Model file for the job. Use its own axes, mm. A direction names the side the tool comes from. Coordinates: 2 decimals unless noted, no trailing zeros. Loops run counter-clockwise (first coordinate to the right, second up) from the corner with the lowest first, then second, coordinate; pieces in that order, holes last.
from build123d import *

# Parameters (mm, degrees)
BASE_FLANGE1_DEPTH = 2
SKETCH7_R          = 2
CUT_EXTRUDE1_DEPTH = 2
SKETCH9_R          = 1.9431
CUT_EXTRUDE2_DEPTH = 2


# Sheet-metal steps are written as plain solids
with BuildPart() as part:
    # Sketch2 → Base-Flange1 (new body)
    with BuildSketch(Plane(origin=(0, 0, 0), x_dir=(1, 0, 0), z_dir=(0, 1, 0))):
        with BuildLine():
            Line((-26.055569119, -21.875), (-26.055569119, -46.875))
            Line((-26.055569119, -46.875), (-16.055569119, -46.875))
            Line((-16.055569119, -46.875), (-16.055569119, -21.875))
            Line((-16.055569119, -21.875), (26.055569119, -21.875))
            Line((26.055569119, -21.875), (26.055569119, 8.188046441))
            ThreePointArc((26.055569119, 8.188046441), (21.514872246, 4.669726518), (15.870079226, 5.73406431))
            ThreePointArc((15.870079226, 5.73406431), (10.616247764, 4.133629141), (7, 0))
            ThreePointArc((7, 0), (0, -7), (-7, 0))
            ThreePointArc((-7, 0), (-10.616247764, 4.133629141), (-15.870079226, 5.73406431))
            ThreePointArc((-15.870079226, 5.73406431), (-21.514872246, 4.669726518), (-26.055569119, 8.188046441))
            Line((-26.055569119, 8.188046441), (-26.055569119, -21.875))
        make_face()
    extrude(amount=-BASE_FLANGE1_DEPTH)

    # Sketch7 → Cut-Extrude1 (cut)
    with BuildSketch(Plane(origin=(0, 0, 0), x_dir=(1, 0, 0), z_dir=(0, 1, 0))):
        with Locations(Location((-21.055569119, -40.375, 0), (0, 0, 270))):
            Circle(SKETCH7_R)
        with Locations(Location((-21.055569119, -30.875, 0), (0, 0, 270))):
            Circle(SKETCH7_R)
    extrude(amount=-CUT_EXTRUDE1_DEPTH, mode=Mode.SUBTRACT)

    # Sketch9 → Cut-Extrude2 (cut)
    with BuildSketch(Plane(origin=(0, 0, 0), x_dir=(1, 0, 0), z_dir=(0, 1, 0))):
        with Locations(Location((-7.875283017, -16.875, 0), (0, 0, 270))):
            Circle(SKETCH9_R)
        with Locations(Location((7.875283017, -16.875, 0), (0, 0, 270))):
            Circle(SKETCH9_R)
    extrude(amount=-CUT_EXTRUDE2_DEPTH, mode=Mode.SUBTRACT)


solid = part.part
Q1. Slice it at C-C (z = 37). List the corners of the cut face in (x, y).
Answers:
outline: (-26.06, -2) - (-16.06, -2) - (-16.06, 0) - (-26.06, 0) - close
Q2. Slice it at A-A (z = 1.5). List the corners of the cut face in (x, y).
Answers:
outline: (-26.06, -2) - (-6.84, -2) - (-6.84, 0) - (-26.06, 0) - close; (6.84, -2) - (26.06, -2) - (26.06, 0) - (6.84, 0) - close
Q3. Which spindle directions (+Z, -Z, +X, -X, +Y, -Y) get a long thin tool onto all of the face, cutting with end or side? Do faces 1 (the flat face through (-16.056, -1, 35)), 2 (the cylindrical face through (-7.292, -0.986, 18.728)), 3 (the cylindrical face through (10.682, -0.986, -4.176)). Say none if no direction does.
Answers:
face 1: +Z, +X, +Y, -Y
face 2: +Y, -Y
face 3: -Z, +Y, -Y
Q4. Mould opens along X. For faces 4 (the cylindrical face through (7.13, -0.99, 18.67)), 5 (the cylindrical face through (-10.55, -0.99, -4.09)), 6 (the flat face through (-26.056, -1, 19)), 7 (the flat face through (-21, -1, 46.875)) say: +X half, -X half, draft (parallel to the pull), parting line (faces both ways), or undercut.
Answers:
face 4: undercut
face 5: undercut
face 6: -X half
face 7: draft
Q5. Drill centre lines: line 1 (X direction, y = -0.7, z = 17.5); line 2 (X direction, y = -1, z = 15.5); line 3 (X direction, y = -1.65, z = 42.5). Where is each one in solid material? Low to high.
Answers:
line 1: x = -26.06 to -9.72, -6.04 to 6.04, 9.72 to 26.06
line 2: x = -26.06 to -9.25, -6.5 to 6.5, 9.25 to 26.06
line 3: x = -26.06 to -16.06
Q6. Slice it at B-B (y = -0.85). List the corners of the cut face in (x, z) (3 decimals), and give its area (3 significant figures).
Answers:
outline: (-26.056, -8.188) arc R7 cw to (-15.87, -5.734) arc R10 ccw to (-7, 0) arc R7 cw to (7, 0) arc R10 ccw to (15.87, -5.734) arc R7 cw to (26.056, -8.188) - (26.056, 21.875) - (-16.056, 21.875) - (-16.056, 46.875) - (-26.056, 46.875) - close; hole circle Ø4 at (-21.056, 30.875); hole circle Ø4 at (-21.056, 40.375); hole circle Ø3.886 at (-7.875, 16.875); hole circle Ø3.886 at (7.875, 16.875)
area: 1,440 mm2
Q7. Slice it at D-D (x = 0). List the corners of the cut face in (y, z) (3 decimals).
Answers:
outline: (-2, 7) - (0, 7) - (0, 21.875) - (-2, 21.875) - close
Q8. Flat gauge pins, fed straight in: P1, Ø3.5, axis at x = -7.88, z = 16.88, coming from the -Y side; P2, Ø0.6, axis at y = -0.5, z = 31.5, coming from the +X side. Where does each tip first touch, or does it go through?
Answers:
P1: passes through
P2: stops at x = -16.06
